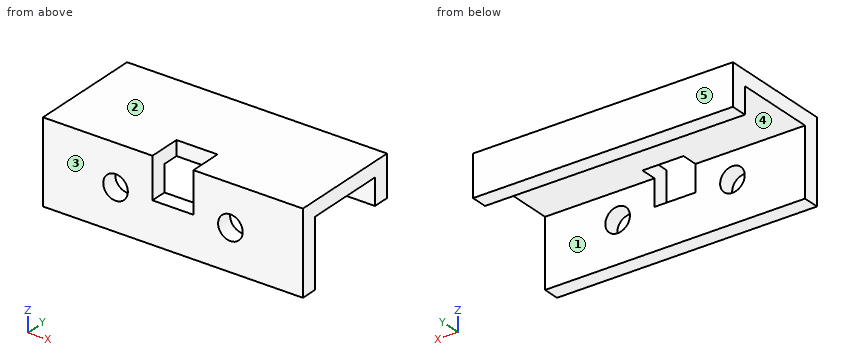
```python
from build123d import *

# Parameters (mm, degrees)
CROQUIS2_W                 = 21.685111185
CROQUIS2_H                 = 10
CROQUIS2_R                 = 1.5
SALIENTE_EXTRUIR1_DEPTH    = 2
CROQUIS3_W                 = 21.685111185
CROQUIS3_H                 = 1.8
SALIENTE_EXTRUIR2_DEPTH    = 10
CORTAR_EXTRUIR1_DEPTH      = 2
CORTAR_EXTRUIR1_DEPTH_BACK = 10
CROQUIS4_W                 = 5
CROQUIS4_H                 = 5
CROQUIS7_W                 = 21.685111185
CROQUIS7_H                 = 5
SALIENTE_EXTRUIR4_DEPTH    = 2
SALIENTE_EXTRUIR5_DEPTH    = 5
SALIENTE_EXTRUIR6_DEPTH    = 5


with BuildPart() as part:
    # Croquis2 → Saliente-Extruir1 (new body)
    with BuildSketch(Plane(origin=(0, 0, 0), x_dir=(1, 0, 0), z_dir=(0, 1, 0))):
        with Locations((10.842555593, 5)):
            Rectangle(CROQUIS2_W, CROQUIS2_H)
        with Locations(Location((3.842555592, 5, 0), (0, 0, 270))):
            Circle(CROQUIS2_R, mode=Mode.SUBTRACT)
        with Locations(Location((17.842555592, 5, 0), (0, 0, 270))):
            Circle(CROQUIS2_R, mode=Mode.SUBTRACT)
    extrude(amount=SALIENTE_EXTRUIR1_DEPTH)

    # Croquis3 → Saliente-Extruir2 (add)
    with BuildSketch(Plane(origin=(0, 2, 0), x_dir=(1, 0, 0), z_dir=(0, 1, 0))):
        with Locations((10.842555593, 0.9)):
            Rectangle(CROQUIS3_W, CROQUIS3_H)
    extrude(amount=SALIENTE_EXTRUIR2_DEPTH)

    # Croquis4 → Cortar-Extruir1 (cut, two sides: drawn at the far end of the back side and taken through both)
    with BuildSketch(Plane(origin=(0, 2, 0), x_dir=(1, 0, 0), z_dir=(0, 1, 0)).offset(-CORTAR_EXTRUIR1_DEPTH_BACK)):
        with Locations((10.842555592, 2.5)):
            Rectangle(CROQUIS4_W, CROQUIS4_H)
    extrude(amount=CORTAR_EXTRUIR1_DEPTH + CORTAR_EXTRUIR1_DEPTH_BACK, mode=Mode.SUBTRACT)

    # Croquis7 → Saliente-Extruir4 (add)
    with BuildSketch(Plane(origin=(0, 12, 0), x_dir=(1, 0, 0), z_dir=(0, 1, 0))):
        with Locations((10.842555593, 2.5)):
            Rectangle(CROQUIS7_W, CROQUIS7_H)
    extrude(amount=SALIENTE_EXTRUIR4_DEPTH)

    # Croquis8 → Saliente-Extruir5 (add)
    with BuildSketch(Plane.ZY):
        Polygon((-10, 0), (0, 0), (0, 14), (-5, 14), (-5, 12), (-1.8, 12), (-1.8, 2), (-10, 2), align=None)
    extrude(amount=SALIENTE_EXTRUIR5_DEPTH)

    # Croquis9 → Saliente-Extruir6 (add)
    with BuildSketch(Plane(origin=(21.685111185, 0, 0), x_dir=(0, 0, -1), z_dir=(1, 0, 0))):
        Polygon((0, 0), (10, 0), (10, 2), (1.8, 2), (1.8, 12), (5, 12), (5, 14), (0, 14), align=None)
    extrude(amount=SALIENTE_EXTRUIR6_DEPTH)


solid = part.part
```
Source: CAD feature listing. Evaluate the final solid. Frame: model axes, mm. Face numbers are marked on the shaded views. A direction names the side the tool comes from. Round coordinates to 2 decimals unless told otherwise and drop trailing zeros. Loops run counter-clockwise (first coordinate to the right, second up) from the corner with the lowest first, then second, coordinate; pieces in that order, holes last.
(1) Section query D-D (y = 6.5). Output: boundary loops of the cut face in (x, z).
From the geometry:
outline: (-5, -1.8) - (26.69, -1.8) - (26.69, 0) - (-5, 0) - close
(2) Access query for the marked faces 4 and 5. Directions: +Z, -Z, +X, -X, +Y, -Y. A direction counts if a zero-diameter tool reaches every point of the face in a straight line with its end or side. Return the directions, or none.
From the geometry:
face 4: -Z, +X, -X
face 5: +Z, -Z, +X, -X, +Y
(3) Section query A-A (x = -2). Output: boundary loops of the cut face in (y, z).
From the geometry:
outline: (0, -10) - (2, -10) - (2, -1.8) - (12, -1.8) - (12, -5) - (14, -5) - (14, 0) - (0, 0) - close
(4) Section query C-C (x = 5). Output: boundary loops of the cut face in (y, z), and give its area (3 significant figures).
From the geometry:
outline: (0, -10) - (2, -10) - (2, -5.95) - (0, -5.95) - close; (0, -4.05) - (2, -4.05) - (2, -1.8) - (12, -1.8) - (12, -5) - (14, -5) - (14, 0) - (0, 0) - close
area: 44.2 mm2
(5) Material intervals for probe 1 along X at (y, z) = (1.5, -1); probe 2 along Y at (x, z) = (-2.5, -4.75); probe 3 along Z at (x, y) = (23, 6.75), sorted ascending.
From the geometry:
probe 1: x = -5 to 8.34, 13.34 to 26.69
probe 2: y = 0 to 2, 12 to 14
probe 3: z = -1.8 to 0
(6) Contact query for flat-ended pins moving along their axis: pin 1 Ø4 at (x, z) = (3, -8.5) entering from +Y; pin 2 Ø8 at (x, y) = (18.5, 9.5) entering from -Z; pin 3 Ø3 at (x, y) = (0, 2.5) entering from +Z; pin 4 Ø3 at (x, y) = (17.5, 4) entering from -Z. Output: stop coordinate, or through.
From the geometry:
pin 1: stops at y = 2
pin 2: stops at z = -5
pin 3: stops at z = 0
pin 4: stops at z = -1.8
(7) Section query B-B (z = -6). Output: boundary loops of the cut face in (x, y).
From the geometry:
outline: (-5, 0) - (2.72, 0) - (2.72, 2) - (-5, 2) - close; (4.96, 0) - (16.72, 0) - (16.72, 2) - (4.96, 2) - close; (18.96, 0) - (26.69, 0) - (26.69, 2) - (18.96, 2) - close
(8) Pull-direction query (Y, two-part tool) for the marked faces 1, 2 and 3; classes: +Y half, -Y half, draft (parallel to the pull), parting line (faces both ways), or undercut.
From the geometry:
face 1: undercut
face 2: draft
face 3: -Y half
